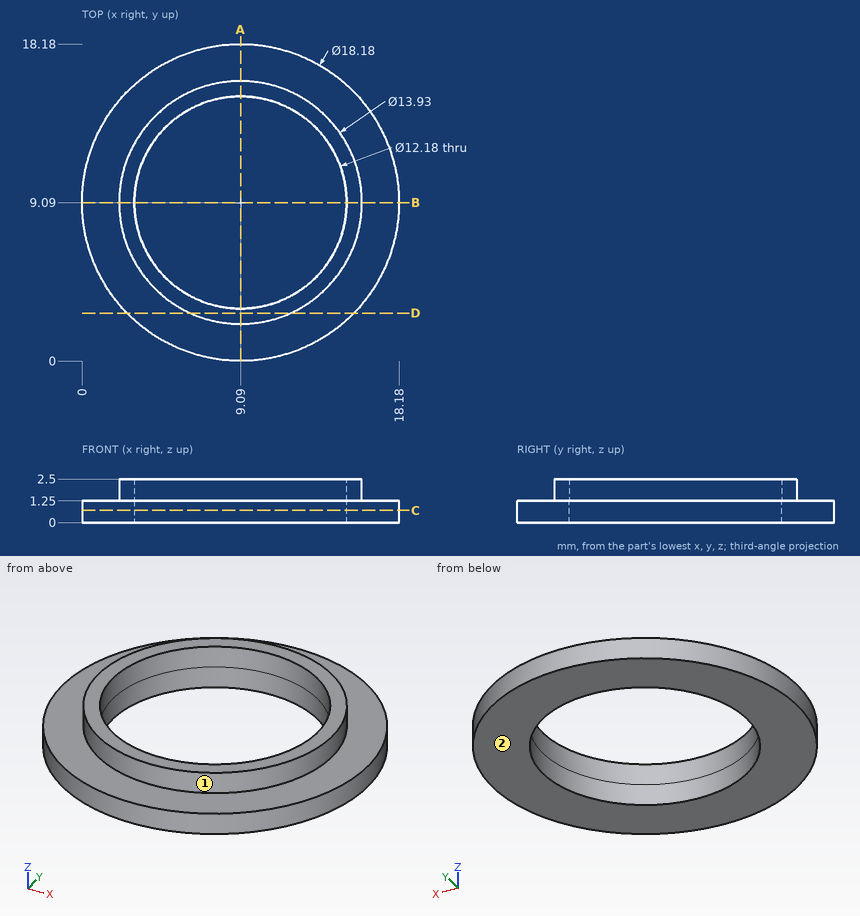
The figure shows three views and two pictorial views of one solid part (mm, origin at its lowest corner). Answer the questions. A direction names the side the tool comes from. Give positions to 0.01 mm unless a question says otherwise; leave off trailing zeros. Write each loop counter-clockwise with the first axis right and the second up, starting at its lowest first coordinate (ties: lowest second). Pieces come first, ordered by that corner, then holes. Notation, with made-up numbers: (-10.5, 42.25) - (1.5, 42.25) arc R11 ccw to (1.5, 58.25) - close; hole circle Ø10 at (80.5, 7.5). An arc over 180 degrees is marked (long way). Use one line per item in the form item = value.
1. For the marked faces 1 and 2, determine the directions among +Z, -Z, +X, -X, +Y, -Y from which every point of the face is accessible in a straight line to the end or side of a thin tool.
Filled in:
face_1 = +Z
face_2 = -Z, +X, -X, +Y, -Y
2. A cutting plane is placed at C-C (z = 0.7). Write down the section's boundary in (x, y).
Filled in:
outline = circle Ø18.18 at (9.09, 9.09); hole circle Ø12.18 at (9.09, 9.09)
3. A cutting plane is placed at D-D (y = 2.75). Write down the section's boundary in (x, z).
Filled in:
outline = (2.58, 0) - (15.6, 0) - (15.6, 1.25) - (11.97, 1.25) - (11.97, 2.5) - (6.21, 2.5) - (6.21, 1.25) - (2.58, 1.25) - close
4. Each of these flat-tipped pins is pushed along its axis until it touches: pin 1 Ø7.5 at (x, y) = (9.09, 9.09) entering from -Z; pin 2 Ø1 at (x, z) = (13, 1) entering from -Y; pin 3 Ø1.5 at (y, z) = (12.5, 1.5) entering from +X; pin 4 Ø1 at (y, z) = (2.5, 2) entering from +X. Where does it stop, or does it pass through?
Filled in:
pin_1 = through
pin_2 = 0.66
pin_3 = 17.77
pin_4 = 12.47
5. Consider L1, parallel to Y at x = 9.09, z = 2.2 (3 decimals); L2, parallel to Y at x = 9.09, z = 0.75; L3, parallel to Z at x = 14, y = 16. Determine where each line is inside the solid, lowest interval first.
Filled in:
L1 = 2.125 to 3, 15.18 to 16.055
L2 = 0 to 3, 15.18 to 18.18
L3 = 0 to 1.25
6. A cutting plane is placed at A-A (x = 9.09). Write down the section's boundary in (y, z) (3 decimals).
Filled in:
outline = (0, 0) - (3, 0) - (3, 2.5) - (2.125, 2.5) - (2.125, 1.25) - (0, 1.25) - close; (15.18, 0) - (18.18, 0) - (18.18, 1.25) - (16.055, 1.25) - (16.055, 2.5) - (15.18, 2.5) - close
